Work out the finished part from the listing and answer in its coordinate system (mm). Face numbers are marked on the shaded views. A direction names the side the tool comes from. Give positions to 0.01 mm unless a question says otherwise; leave off trailing zeros. Order: outer loops, then holes, each group sorted by start corner. A loop starts at its lowest first (then second) coordinate and runs counter-clockwise, first axis right, second up. Notation, with made-up numbers: M 84.5,78 L 112.5,78 A17 cw 112.5,89 Z; hole C 78,85 d3. An arc over 180 degrees is marked long. One line per item, written item: value.
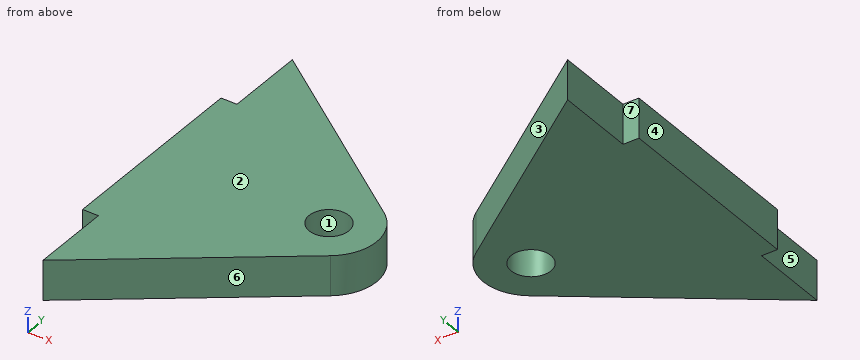
from build123d import *

# Parameters (mm, degrees)
SZKIC1_R                    = 2.5
SZKIC1_W                    = 2
SZKIC1_H                    = 25
DODANIE_WYCI_GNI_CIE1_DEPTH = 5


with BuildPart() as part:
    # Szkic1 → Dodanie-wyciągnięcie1 (new body)
    with BuildSketch(Plane.XY):
        with BuildLine():
            ThreePointArc((214.351594971, 216.879691308), (216.781303051, 212.057553235), (214.351594971, 207.235415161))
            Line((214.351594971, 207.235415161), (190.475370577, 189.557553235))
            Line((190.475370577, 189.557553235), (190.475370577, 199.557553235))
            Line((190.475370577, 199.557553235), (190.475370577, 224.557553235))
            Line((190.475370577, 224.557553235), (190.475370577, 234.557553235))
            Line((190.475370577, 234.557553235), (214.351594971, 216.879691308))
        make_face()
        with Locations((210.781303051, 212.057553235)):
            Circle(SZKIC1_R, mode=Mode.SUBTRACT)
        with Locations((189.475370577, 212.057553235)):
            Rectangle(SZKIC1_W, SZKIC1_H)
    extrude(amount=DODANIE_WYCI_GNI_CIE1_DEPTH)


solid = part.part
(1) Determine the mould class of the marked faces 1, 2, 3 and 4 for opening direction X: pulls with the +X half, pulls with the -X half, needs draft (parallel to the pull), parting line crosses it, or undercut.
Findings:
face 1: undercut
face 2: needs draft
face 3: pulls with the +X half
face 4: pulls with the -X half
(2) Find the intervals of material crossed by probe 1 along Y at (x, z) = (210.75, 1.5); probe 2 along X at (y, z) = (210.5, 2.2); probe 3 along Y at (x, z) = (209.5, 2.6), in increasing order. Write a range as from..to.
Findings:
probe 1: y = 204.57..209.56, 214.56..219.55
probe 2: x = 188.48..208.83, 212.74..216.58
probe 3: y = 203.64..209.91, 214.2..220.47
(3) Given P1, Ø2, axis at y = 195.5, z = 1, coming from the +X side; P2, Ø1, axis at x = 189.5, z = 2.5, coming from the +Y side; P3, Ø1.5, axis at x = 193, z = 1, coming from the -Y side, each flat-ended and moving along its own axis, determine where each tip first touches the part or whether it passes through.
Findings:
P1: stops at x = 199.85
P2: stops at y = 224.56
P3: stops at y = 190.87
(4) Section A-A, the plane x = 209.25 is taken. Give the vertices of the cut face in (y, z).
Findings:
outline: M 203.46,0 L 210.08,0 L 210.08,5 L 203.46,5 Z; M 214.03,0 L 220.66,0 L 220.66,5 L 214.03,5 Z
(5) Section B-B, the plane z = 1 is taken. Give the vertices of the cut face in (x, y).
Findings:
outline: M 188.48,199.56 L 190.48,199.56 L 190.48,189.56 L 214.35,207.24 A6 ccw 214.35,216.88 L 190.48,234.56 L 190.48,224.56 L 188.48,224.56 Z; hole C 210.78,212.06 d5
(6) Which of the six approach directions +Z, -Z, +X, -X, +Y, -Y give full straight-line access (tool end or side, diameter ignored) to the marked faces 5, 6 and 7?
Findings:
face 5: +Z, -Z, -X, -Y
face 6: +Z, -Z, +X, -Y
face 7: +Z, -Z, -X, +Y
(7) Section C-C, the plane x = 213.75 is taken. Give the vertices of the cut face in (y, z), then the cut area to 3 significant figures.
Findings:
outline: M 206.79,0 L 217.33,0 L 217.33,5 L 206.79,5 Z
area: 52.7 mm^2
(8) Section D-D, the plane y = 227.5 is taken. Give the vertices of the cut face in (x, z).
Findings:
outline: M 190.48,0 L 200.01,0 L 200.01,5 L 190.48,5 Z
